Read the model definition and answer for the solid it produces. Units are mm, in the model's axes. A direction names the side the tool comes from. Give positions to 0.01 mm unless a question says otherwise; leave off trailing zeros. Order: outer loops, then holes, each group sorted by start corner. A loop starts at its lowest first (then second) coordinate and runs counter-clockwise, first axis right, second up. Notation, with made-up numbers: (-15.5, -0.5) - (0.5, -0.5) arc R26 ccw to (0.5, 19.5) - close; hole circle Ø7 at (-2, 13.5). An arc over 180 degrees is marked (long way). Write each question's results on one line, items separated by ' | '. Start each with the question number.
Q1. Find the intervals of material crossed by line 1 along Z through (x, y) = (3.5, 1.6); line 2 along X through (y, z) = (6.75, -6.75); line 3 along X through (y, z) = (7, -3.25), in increasing order. Write a range as from..to.
Q2. Find section A-A on x = 3.5. Give the vertices of the cut face in (y, z).
Q3. Find section C-C on x = 0. Give the vertices of the cut face in (y, z), and give its area (3 significant figures).
Q4. A tool of negligible diameter and unlimited length cuts with its end or side. For faces 5 (the face through (-1, 3.6, -2.3)), 6 (the face through (-5, 4, -7)), 7 (the face through (-0.1, 5.2, -2.915)), from which of +Z, -Z, +X, -X, +Y, -Y can it reach the whole face along a straight path? Write none if from no direction.
Q5. For a pull along X with two mould halves and no side action, classify faces 1 (the face through (5, 4, -7)), 2 (the face through (-7.5, 1, 1)), 3 (the face through (0, 4, -11.915)), 4 (the face through (3.153, 1.479, 2.647)) as +X half, -X half, draft (parallel to the pull), parting line (faces both ways), or undercut.
Q6. Find section D-D on y = 0.5. Give the vertices of the cut face in (x, z).
Q7. Find section B-B on z = -8. Give the vertices of the cut face in (x, y).
Q8. Flat-ended cylindrical pins translate along their axes: P1, Ø1.2, axis at x = -7, y = 2, coming from the -Z side; P2, Ø3.5, axis at x = 3.5, z = 1.08, coming from the +Y side; P3, Ø1.5, axis at y = 3.5, z = -10, coming from the -X side. Find the tip coordinate at first contact, or state that the pin passes through.
from build123d import *

# Parameters (mm, degrees)
SKETCH1_W           = 15
SKETCH1_H           = 8
SKETCH1_R           = 1.6
BOSS_EXTRUDE1_DEPTH = 3
SKETCH2_W           = 10
SKETCH2_H           = 9
SKETCH2_R           = 2.5
BOSS_EXTRUDE2_DEPTH = 7.5
BOSS_EXTRUDE3_DEPTH = 1


with BuildPart() as part:
    # Sketch1 → Boss-Extrude1 (new body)
    with BuildSketch(Plane(origin=(0, 0, 0), x_dir=(1, 0, 0), z_dir=(0, 1, 0))):
        with Locations((0, -1.0848967)):
            Rectangle(SKETCH1_W, SKETCH1_H)
        with Locations((-3.5, -1.0848967)):
            Circle(SKETCH1_R, mode=Mode.SUBTRACT)
        with Locations((3.5, -1.0848967)):
            Circle(SKETCH1_R, mode=Mode.SUBTRACT)
    extrude(amount=BOSS_EXTRUDE1_DEPTH)

    # Sketch2 → Boss-Extrude2 (add)
    with BuildSketch(Plane(origin=(0, 0, 0), x_dir=(1, 0, 0), z_dir=(0, 1, 0))):
        with Locations((0, 7.4151033)):
            Rectangle(SKETCH2_W, SKETCH2_H)
        with Locations((0, 6.9151033)):
            Circle(SKETCH2_R, mode=Mode.SUBTRACT)
    extrude(amount=BOSS_EXTRUDE2_DEPTH)

    # Sketch4 → Boss-Extrude3 (add, symmetric)
    with BuildSketch(Plane(origin=(0, 0, 0), x_dir=(0, 0, -1), z_dir=(1, 0, 0))):
        Polygon((2.9151033, 5), (0.9151033, 3), (2.9151033, 3), align=None)
    extrude(amount=BOSS_EXTRUDE3_DEPTH, both=True)


solid = part.part
Working result:
1) line 1: -11.92..-0.52, 2.68..5.08 | line 2: -5..-2.49, 2.49..5 | line 3: -5..5
2) outline: (0, -11.92) - (7.5, -11.92) - (7.5, -2.92) - (3, -2.92) - (3, -0.52) - (0, -0.52) - close; (0, 2.68) - (3, 2.68) - (3, 5.08) - (0, 5.08) - close
3) outline: (0, -11.92) - (7.5, -11.92) - (7.5, -9.42) - (0, -9.42) - close; (0, -4.42) - (7.5, -4.42) - (7.5, -2.92) - (5, -2.92) - (3, -0.92) - (3, 5.08) - (0, 5.08) - close | area: 56.0 mm²
4) face 5: +Z, -X, +Y | face 6: -Z, -X, +Y, -Y | face 7: +Z, +Y
5) face 1: +X half | face 2: -X half | face 3: draft | face 4: undercut
6) outline: (-7.5, -2.92) - (-5, -2.92) - (-5, -11.92) - (5, -11.92) - (5, -2.92) - (7.5, -2.92) - (7.5, 5.08) - (-7.5, 5.08) - close; hole circle Ø3.2 at (-3.5, 1.08); hole circle Ø5 at (0, -6.92); hole circle Ø3.2 at (3.5, 1.08)
7) outline: (-5, 0) - (-2.25, 0) - (-2.25, 7.5) - (-5, 7.5) - close; (2.25, 0) - (5, 0) - (5, 7.5) - (2.25, 7.5) - close
8) P1: z = -2.92 | P2: y = 3 | P3: x = -5
